Build history of the part. All positions in model axes, mm. Face numbers are marked on the shaded views. A direction names the side the tool comes from. Round coordinates to 2 decimals unless told otherwise and drop trailing zeros. Answer as CSV lines item,"result". Start each with the question number.
```python
from build123d import *

# Parameters (mm, degrees)
F1_DEPTH = 155
F2_START = 15
F2_DEPTH = 125
F3_R     = 4
F4_W     = 30.3553390593
F4_H     = 44
F5_DEPTH = 215
F4_W_2   = 15
F4_H_2   = 35
F6_DEPTH = 180
F7_START = 5
F7_DEPTH = 145
F8_R     = 5


with BuildPart() as f1:
    # F0 (on Top) → F1 (new body)
    with BuildSketch(Plane.XY):
        Polygon((73, -25), (100, 2), (100, 40), (-97, 40), (-97, -25), align=None)
        Polygon((95, 35), (95, 4.0710678119), (70.9289321881, -20), (-92, -20), (-92, 35), align=None, mode=Mode.SUBTRACT)
        Polygon((70.9289321881, -20), (95, 4.0710678119), (95, 35), (-92, 35), (-92, -20), align=None)
    extrude(amount=F1_DEPTH)

    # F0 (on Top) → F2 (join)
    with BuildSketch(Plane.XY.offset(F2_START)):
        Polygon((-114.6776695297, -28.5355339059), (-103.2132034356, -40), (79.6446609407, -40), (115, -4.6446609407), (115, 55), (-97, 55), (-114.6776695297, 37.3223304703), align=None)
        Polygon((100, 40), (100, 2), (73, -25), (-97, -25), (-97, 40), align=None, mode=Mode.SUBTRACT)
    extrude(amount=F2_DEPTH)

    # F3
    f3_edges = [f1.edges().sort_by_distance(p)[0] for p in [
        (97.32233, -22.32233, 140),
        (115, 25.17767, 140),
        (9, 55, 140),
        (-105.838835, 46.161165, 140),
        (-114.67767, 4.393398, 140),
        (-108.945436, -34.267767, 140),
        (-11.784271, -40, 140),
        (100, 21, 140),
        (86.5, -11.5, 140),
        (-12, -25, 140),
        (-97, 7.5, 140),
        (1.5, 40, 140),
        (97.32233, -22.32233, 15),
        (115, 25.17767, 15),
        (9, 55, 15),
        (-105.838835, 46.161165, 15),
        (-114.67767, 4.393398, 15),
        (-108.945436, -34.267767, 15),
        (-11.784271, -40, 15),
        (100, 21, 15),
        (86.5, -11.5, 15),
        (-12, -25, 15),
        (-97, 7.5, 15),
        (1.5, 40, 15),
    ]]
    fillet(f3_edges, radius=F3_R)

    # F4 (on face) → F5 (cut)
    with BuildSketch(Plane.YZ.offset(115)):
        Polygon((31, 121), (31, 130), (-4.6446609407, 130), (-4.6446609407, 86), (31, 86), align=None)
        with Locations((-19.8223304703, 108)):
            Rectangle(F4_W, F4_H)
        with Locations((-19.8223304703, 47)):
            Rectangle(F4_W, F4_H)
        Polygon((31, 69), (-4.6446609407, 69), (-4.6446609407, 25), (31, 25), (31, 34), align=None)
    extrude(amount=-F5_DEPTH, mode=Mode.SUBTRACT)

    # F4 (on face) → F6 (cut)
    with BuildSketch(Plane.YZ.offset(115)):
        with Locations((38.5, 51.5)):
            Rectangle(F4_W_2, F4_H_2)
        with Locations((38.5, 103.5)):
            Rectangle(F4_W_2, F4_H_2)
    extrude(amount=-F6_DEPTH, mode=Mode.SUBTRACT)

    # F0 (on Top) → F7 (cut)
    with BuildSketch(Plane.XY.offset(F7_START)):
        Polygon((70.9289321881, -20), (95, 4.0710678119), (95, 35), (-92, 35), (-92, -20), align=None)
    extrude(amount=F7_DEPTH, mode=Mode.SUBTRACT)

    # F8
    f8_edges = [f1.edges().sort_by_distance(p)[0] for p in [
        (105, 31, 121),
        (105, 31, 34),
        (-100, 31, 108),
        (-100, -2, 130),
        (-100, -35, 108),
        (-100, -2, 86),
        (-100, -35, 47),
        (-100, -2, 25),
        (-100, 31, 47),
        (-100, -2, 69),
        (82.964466, -7.964466, 5),
        (95, 19.535534, 5),
        (1.5, 35, 5),
        (-92, 7.5, 5),
        (-10.535534, -20, 5),
        (82.964466, -7.964466, 150),
        (95, 19.535534, 150),
        (1.5, 35, 150),
        (-92, 7.5, 150),
        (-10.535534, -20, 150),
        (25, 46, 86),
        (25, 46, 121),
        (115, 46, 103.5),
        (-65, 46, 103.5),
        (25, 46, 34),
        (25, 46, 69),
        (115, 46, 51.5),
        (-65, 46, 51.5),
        (115, 38.5, 34),
        (115, 20.67767, 69),
        (115, 20.67767, 86),
        (115, 38.5, 121),
    ]]
    fillet(f8_edges, radius=F8_R)


solid = f1.part
```
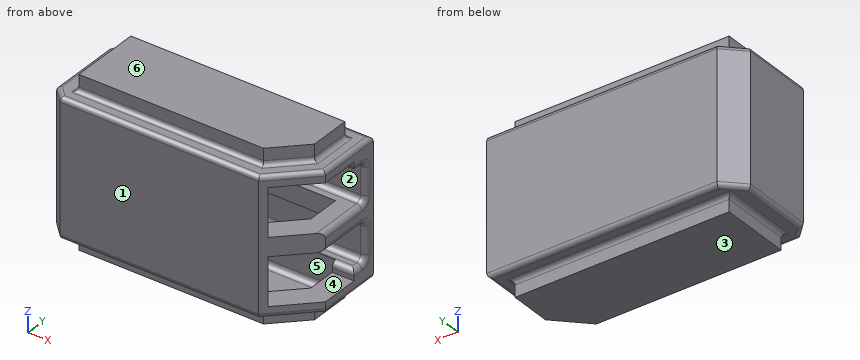
Q1. Pin check, flat tips, straight feed: pin 1 Ø5.5 at (x, z) = (43.5, 150) entering from +Y; pin 2 Ø9 at (x, z) = (-30, 152) entering from -Y; pin 3 Ø3 at (x, z) = (109.5, 28) entering from -Y. Stop position of each tip, or through.
Q2. Tool access for the marked faces 4, 5 and 6: list every direction of +Z, -Z, +X, -X, +Y, -Y with a clear straight run to the whole face (end or side of a thin tool).
Q3. Wall check: probe 1 along Z at (x, y) = (-18, -31.5); probe 2 along Z at (x, y) = (85, -8.5); probe 3 along Y at (x, z) = (18.5, 110). Give the ranges that are in metal, low to high. Write a range as [from, to].
Q4. Two-plate mould, pull along Z, no slides. Class the marked faces 1, 2 and 3: released by +Z, released by -Z, zero draft, split by the parting line, or undercut.
Reported:
1,pin 1,"stops at y = 40"
1,pin 2,"stops at y = -25"
1,pin 3,"stops at y = 31"
2,face 4,"+X"
2,face 5,"none"
2,face 6,"+Z, +X, -X, +Y, -Y"
3,probe 1,"z = [15, 25], [69, 86], [130, 140]"
3,probe 2,"z = [0, 25], [69, 86], [130, 155]"
3,probe 3,"y = [-40, -35], [46, 55]"
4,face 1,"zero draft"
4,face 2,"undercut"
4,face 3,"released by -Z"
